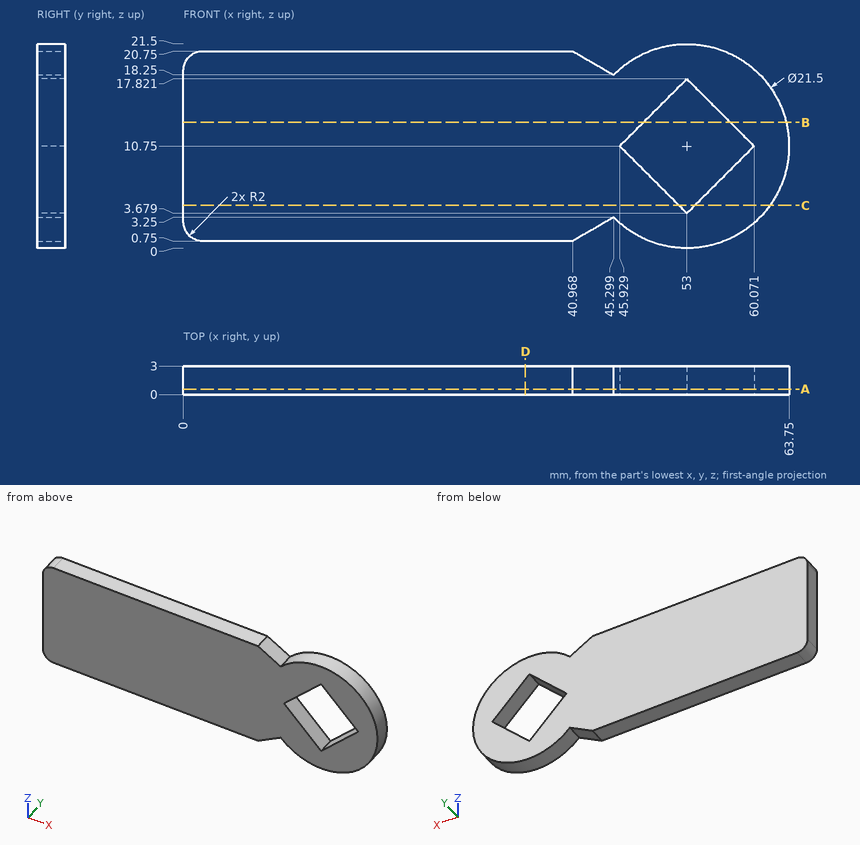
Here's the drawing with two shaded views (mm, measured from the low corner). I have some questions. Give positions to 0.01 mm unless a question says otherwise; leave off trailing zeros. Loops run counter-clockwise (first coordinate to the right, second up) from the corner with the lowest first, then second, coordinate; pieces in that order, holes last. Notation, with made-up numbers: (-31.5, -27.75) - (4.5, -27.75) arc R28 ccw to (4.5, 10.25) - close; hole circle Ø5 at (15, 38.5). An arc over 180 degrees is marked (long way). One line per item, written item: value.
(1) If we section it at C-C, the plane z = 4.5: List the corners of the cut face in (x, y) for me, plus the area to 3 significant figures.
Verdict:
outline: (0, 0) - (52.18, 0) - (52.18, 3) - (0, 3) - close; (53.82, 0) - (61.75, 0) - (61.75, 3) - (53.82, 3) - close
area: 180 mm^2
(2) If we section it at D-D, the plane x = 36: List the corners of the cut face in (y, z) for me.
Verdict:
outline: (0, 0.75) - (3, 0.75) - (3, 20.75) - (0, 20.75) - close
(3) I need wall thicknesses on line 1 along Z through (x, y) = (9, 2.7); line 2 along Z through (x, y) = (51, 1.25) (1 decimal); line 3 along X through (y, z) = (2.6, 14.75). Which ranges of each line are inside material? Lowest first, please.
Verdict:
line 1: 0.75 to 20.75
line 2: 0.2 to 5.7, 15.8 to 21.3
line 3: 0 to 49.93, 56.07 to 62.98
(4) If we section it at B-B, the plane z = 13.25: List the corners of the cut face in (x, y) for me (1 decimal).
Verdict:
outline: (0, 0) - (48.4, 0) - (48.4, 3) - (0, 3) - close; (57.6, 0) - (63.5, 0) - (63.5, 3) - (57.6, 3) - close
(5) If we section it at A-A, the plane y = 0.6: List the corners of the cut face in (x, z) for me, plus the area to 4 significant figures.
Verdict:
outline: (0, 2.75) arc R2 ccw to (2, 0.75) - (40.97, 0.75) - (45.3, 3.25) arc R10.75 ccw (long way) to (45.3, 18.25) - (40.97, 20.75) - (2, 20.75) arc R2 ccw to (0, 18.75) - close; hole (45.93, 10.75) - (53, 3.68) - (60.07, 10.75) - (53, 17.82) - close
area: 1,125 mm^2
(6) I'm going to push flat-ended pins straight in: pin 1 (0.9 mm diameter, centred on x = 24, y = 1, fed in from -Z); pin 2 (1.5 mm diameter, centred on x = 30, y = 1.5, fed in from +Z). Where does each tip first touch, or does it pass through?
Verdict:
pin 1: z = 0.75
pin 2: z = 20.75
